Can you work these out from the model? Positions are in its coordinate system, mm. A direction names the side the tool comes from. Give positions to 0.01 mm unless a question says otherwise; leave off trailing zeros. Write each loop counter-clockwise with the first axis right and the second up, starting at its lowest first coordinate (ties: lowest second). Pieces come first, ordered by that corner, then holes.
```python
from build123d import *

# Parameters (mm, degrees)
F0_R     = 4.426475661
F1_DEPTH = 1.5875
F3_DEPTH = 3.1760001


with BuildPart() as f1:
    # F0 (on Front) → F1 (new body, symmetric)
    with BuildSketch(Plane.XZ):
        Polygon((54.356, -63.5), (63.5, -63.5), (63.5, -12.7), (58.658125, -12.7), (58.658125, -14.89075), (55.88, -14.89075), (55.88, -12.7), (50.8, -12.7), (50.8, -9.144), (55.88, -9.144), (55.88, -6.95325), (58.658125, -6.95325), (58.658125, -9.144), (63.5, -9.144), (63.5, 38.1), (58.658125, 38.1), (58.658125, 35.90925), (55.88, 35.90925), (55.88, 38.1), (50.8, 38.1), (50.8, 41.656), (55.88, 41.656), (55.88, 43.84675), (58.658125, 43.84675), (58.658125, 41.656), (63.5, 41.656), (63.5, 63.5), (-63.5, 63.5), (-63.5, 41.656), (-58.658125, 41.656), (-58.658125, 43.84675), (-55.88, 43.84675), (-55.88, 41.656), (-50.8, 41.656), (-50.8, 38.1), (-55.88, 38.1), (-55.88, 35.90925), (-58.658125, 35.90925), (-58.658125, 38.1), (-63.5, 38.1), (-63.5, -9.144), (-58.658125, -9.144), (-58.658125, -6.95325), (-55.88, -6.95325), (-55.88, -9.144), (-50.8, -9.144), (-50.8, -12.7), (-55.88, -12.7), (-55.88, -14.89075), (-58.658125, -14.89075), (-58.658125, -12.7), (-63.5, -12.7), (-63.5, -63.5), (-50.8, -63.5), (-50.8, -58.658125), (-52.99075, -58.658125), (-52.99075, -55.88), (-50.8, -55.88), (-50.8, -50.8), (-47.244, -50.8), (-47.244, -55.88), (-45.05325, -55.88), (-45.05325, -58.658125), (-47.244, -58.658125), (-47.244, -63.5), (0, -63.5), (0, -58.658125), (-2.19075, -58.658125), (-2.19075, -55.88), (0, -55.88), (0, -50.8), (3.556, -50.8), (3.556, -55.88), (5.74675, -55.88), (5.74675, -58.658125), (3.556, -58.658125), (3.556, -63.5), (50.8, -63.5), (50.8, -58.658125), (48.60925, -58.658125), (48.60925, -55.88), (50.8, -55.88), (50.8, -50.8), (54.356, -50.8), (54.356, -55.88), (56.54675, -55.88), (56.54675, -58.658125), (54.356, -58.658125), align=None)
        with BuildLine():
            ThreePointArc((-32.5203218701, 31.7733835659), (-40.4536461397, 53.6985968598), (-19.05, 44.45))
            ThreePointArc((-19.05, 44.45), (-21.1583387907, 37.4423818007), (-26.7833406026, 32.7614460077))
            ThreePointArc((-26.7833406026, 32.7614460077), (-29.5944538957, 31.9342650638), (-32.5203218701, 31.7733835659))
        make_face(mode=Mode.SUBTRACT)
        with BuildLine():
            add(Edge.make_bspline(
                [(44.45, 0), (44.45, 3.6661742094), (41.275, 7.0704788323)],
                knots=[0, 0, 0, 0.3802512067, 0.3802512067, 0.3802512067], degree=2, weights=[1, 0.9819805061, 1]))
            add(Edge.make_bspline(
                [(-41.275, 7.0704788323), (-61.2505208253, -14.3477126296), (-8.4002604126, -18.7067286405), (44.45, -23.0657446513), (44.45, 0)],
                knots=[2.7613414469, 2.7613414469, 2.7613414469, 4.522263377, 4.522263377, 6.2831853072, 6.2831853072, 6.2831853072], degree=2, weights=[1, 0.6367957928, 1, 0.6367957928, 1]))
            add(Edge.make_bspline(
                [(-34.925, 11.7841313872), (-38.89375, 9.6237072996), (-41.275, 7.0704788323)],
                knots=[2.4746463091, 2.4746463091, 2.4746463091, 2.7613414469, 2.7613414469, 2.7613414469], degree=2, weights=[1, 0.9897433186, 1]))
            add(Edge.make_bspline(
                [(34.925, 11.7841313872), (0, 30.7958633586), (-34.925, 11.7841313872)],
                knots=[0.6669463445, 0.6669463445, 0.6669463445, 2.4746463091, 2.4746463091, 2.4746463091], degree=2, weights=[1, 0.6185895741, 1]))
            add(Edge.make_bspline(
                [(41.275, 7.0704788323), (38.89375, 9.6237072996), (34.925, 11.7841313872)],
                knots=[0.3802512067, 0.3802512067, 0.3802512067, 0.6669463445, 0.6669463445, 0.6669463445], degree=2, weights=[1, 0.9897433186, 1]))
        make_face(mode=Mode.SUBTRACT)
        with Locations((0, 31.75)):
            Circle(F0_R, mode=Mode.SUBTRACT)
        with BuildLine():
            ThreePointArc((38.02746706, 56.2953220395), (42.727564203, 51.6414036807), (44.45, 45.2552401869))
            ThreePointArc((44.45, 45.2552401869), (22.3090487849, 36.7606277676), (33.0864661175, 57.8847238785))
            ThreePointArc((33.0864661175, 57.8847238785), (35.639028691, 57.3451308333), (38.02746706, 56.2953220395))
        make_face(mode=Mode.SUBTRACT)
        with BuildLine():
            Line((38.1654474814, 54.2776674622), (38.02746706, 56.2953220395))
            ThreePointArc((38.02746706, 56.2953220395), (35.639028691, 57.3451308333), (33.0864661175, 57.8847238785))
            Line((33.0864661175, 57.8847238785), (32.0418357229, 55.2197649229))
            ThreePointArc((32.0418357229, 55.2197649229), (34.5150625993, 50.9229662535), (38.1654474814, 54.2776674622))
        make_face()
        with BuildLine():
            Line((-32.5203218701, 33.4118034209), (-32.5203218701, 31.7733835659))
            ThreePointArc((-32.5203218701, 31.7733835659), (-29.5944538957, 31.9342650638), (-26.7833406026, 32.7614460077))
            Line((-26.7833406026, 32.7614460077), (-26.7833406026, 34.2687429437))
            ThreePointArc((-26.7833406026, 34.2687429437), (-30.3117243032, 38.2580810463), (-32.5203218701, 33.4118034209))
        make_face()
        with BuildLine():
            add(Edge.make_bspline(
                [(-34.925, 11.7841313872), (-38.89375, 9.6237072996), (-41.275, 7.0704788323)],
                knots=[2.4746463091, 2.4746463091, 2.4746463091, 2.7613414469, 2.7613414469, 2.7613414469], degree=2, weights=[1, 0.9897433186, 1]))
            Line((-41.275, 7.0704788323), (-41.275, 0))
            Line((-41.275, 0), (-34.925, 0))
            Line((-34.925, 0), (-34.925, 11.7841313872))
        make_face()
        with BuildLine():
            Line((41.275, 0), (41.275, 7.0704788323))
            add(Edge.make_bspline(
                [(41.275, 7.0704788323), (38.89375, 9.6237072996), (34.925, 11.7841313872)],
                knots=[0.3802512067, 0.3802512067, 0.3802512067, 0.6669463445, 0.6669463445, 0.6669463445], degree=2, weights=[1, 0.9897433186, 1]))
            Line((34.925, 11.7841313872), (34.925, 0))
            Line((34.925, 0), (41.275, 0))
        make_face()
    extrude(amount=F1_DEPTH, both=True)

    # F2 (on face) → F3 (cut, through all)
    with BuildSketch(Plane.XZ.offset(1.5875)):
        Polygon((-53.9152510464, -25.4), (-53.9152510464, -29.21), (-9.1524110914, -29.21), (9.1524110914, -29.21), (54.6370558441, -29.21), (54.6370558441, -25.4), align=None)
        Polygon((9.1524110914, -29.21), (-9.1524110914, -29.21), (-4.5762055457, -33.7862055457), (0, -38.3624110914), (4.5762055457, -33.7862055457), align=None)
        Polygon((0, -38.3624110914), (-4.5762055457, -33.7862055457), (-8.2022583859, -41.7798972868), (0, -45.5005589385), (8.2022583859, -41.7798972868), (4.5762055457, -33.7862055457), align=None)
    extrude(amount=-F3_DEPTH, mode=Mode.SUBTRACT)


solid = f1.part
```
1) Suppose I cut it at B-B on y = 1.05. State how many separate pieces and enclosed holes the cut face has, plus the area to 3 significant figures.
Values follow:
separate pieces: 1
enclosed holes: 5
area: 11,600 mm2
2) Please list where these lines run through material, in increasing order: L1, parallel to X at y = 0.65, z = 44.45; L2, parallel to Z at x = -7.5, y = -0.65; L3, parallel to Z at x = 6, y = 0.1.
Values follow:
L1: x = -63.5 to -44.45, -19.05 to 19.08, 44.42 to 63.5
L2: z = -63.5 to -42.1, -40.23 to -30.86, -25.4 to -18.78, 18.78 to 63.5
L3: z = -63.5 to -42.78, -36.92 to -32.36, -25.4 to -18.88, 18.88 to 63.5
3) Suppose I cut it at A-A on z = -38.5. Write out the boundary of the cut face in (x, y), plus the area to 3 significant figures.
Values follow:
outline: (-63.5, -1.59) - (-6.71, -1.59) - (-6.71, 1.59) - (-63.5, 1.59) - close; (6.71, -1.59) - (63.5, -1.59) - (63.5, 1.59) - (6.71, 1.59) - close
area: 361 mm2
4) For faces 1 (the face through (53, 0, -12.7)), 2 (the face through (-61, 0, 38.1)), 3 (the face through (-32, 0, -29.21)), 4 (the face through (-49, 0, -50.8)), which set-ups out of +Z, -Z, +X, -X, +Y, -Y let a thin tool reach every point of the face, with its end or its side?
Values follow:
face 1: +X, +Y, -Y
face 2: -X, +Y, -Y
face 3: +Y, -Y
face 4: -Z, +Y, -Y
5) If we mould it in two halves opening along X, with no side actions, what happens to faces 5 (the face through (-50.8, 0, 40)), 6 (the face through (-41.275, 0, 4)), 7 (the face through (38, 0, 0)), 8 (the face through (61, 0, 38.1))? For each: +X half, -X half, draft (parallel to the pull), parting line (faces both ways), or undercut.
Values follow:
face 5: -X half
face 6: undercut
face 7: undercut
face 8: draft
